CAD build for the part. Positions are in the model's coordinates, mm. A direction names the side the tool comes from. Round coordinates to 2 decimals unless told otherwise and drop trailing zeros. Write each loop counter-clockwise with the first axis right and the second up, starting at its lowest first coordinate (ties: lowest second). Pieces come first, ordered by that corner, then holes. Notation, with made-up numbers: (53, 41) -> (100, 41) arc R32 ccw to (100, 72) -> close; hole circle Ø11 at (-10.5, 42.25). An arc over 180 degrees is marked (long way). Put each result on its own line as item: value. Start each with the question number.
1. 3-axis set-ups, long thin cutter, end or side, ignore diameter. For faces 1 (the flat face through (1.014, -0.986, 1.724)), 2 (the cylindrical face through (0, 2, -1)): which of +Z, -Z, +X, -X, +Y, -Y reach the whole face in a straight line?
2. Saw through at A-A on z = -0.6. List the corners of the cut face in (x, y), and give its area (3 significant figures).
3. Saw through at B-B on y = -0.5. List the corners of the cut face in (x, z).
4. Saw through at D-D on y = 2.5. List the corners of the cut face in (x, z).
5. Saw through at C-C on x = 0.7. List the corners of the cut face in (y, z).
6. Drill centre lines: line 1 (Y direction, x = -1.65, z = 0.1); line 2 (X direction, y = 1.5, z = -0.5); line 3 (X direction, y = 0.25, z = 0). Where is each one in solid material? Low to high. Write a range as from..to.
7. Flat gauge pins, fed straight in: P1, Ø1, axis at x = -1, y = 4, coming from the +Z side; P2, Ø1, axis at x = -1.5, z = 1, coming from the +Y side; P3, Ø1.5, axis at x = -0.5, z = -1.5, coming from the +Y side. Where does each tip first touch, or does it go through?
from build123d import *

# Parameters (mm, degrees)
F0_R     = 1
F1_DEPTH = 2
F2_R     = 1
F3_DEPTH = 5
F4_DEPTH = 2


with BuildPart() as f1:
    # F0 (on Front) → F1 (new body)
    with BuildSketch(Plane.XZ):
        Polygon((-2, 1.1547005384), (-2, -1.1547005384), (0, -2.3094010768), (2, -1.1547005384), (2, 1.1547005384), (0, 2.3094010768), align=None)
        Circle(F0_R, mode=Mode.SUBTRACT)
        Circle(F0_R)
    extrude(amount=F1_DEPTH)

    # F2 (on face) → F3 (join)
    with BuildSketch(Plane(origin=(0, 0, 0), x_dir=(-1, 0, 0), z_dir=(0, 1, 0))):
        Circle(F2_R)
    extrude(amount=F3_DEPTH)

    # F0 (on Front) → F4 (join)
    with BuildSketch(Plane.XZ):
        Polygon((-2, 1.1547005384), (-2, -1.1547005384), (0, -2.3094010768), (2, -1.1547005384), (2, 1.1547005384), (0, 2.3094010768), align=None)
        Circle(F0_R, mode=Mode.SUBTRACT)
    extrude(amount=F4_DEPTH)


solid = f1.part
Return value:
1. face 1: +Z, +X, +Y, -Y
1. face 2: +Y
2. outline: (-2, -2) -> (2, -2) -> (2, 0) -> (0.8, 0) -> (0.8, 5) -> (-0.8, 5) -> (-0.8, 0) -> (-2, 0) -> close
2. area: 16.0 mm^2
3. outline: (-2, -1.15) -> (0, -2.31) -> (2, -1.15) -> (2, 1.15) -> (0, 2.31) -> (-2, 1.15) -> close
4. outline: circle Ø2 at (0, 0)
5. outline: (-2, -1.91) -> (0, -1.91) -> (0, -0.71) -> (5, -0.71) -> (5, 0.71) -> (0, 0.71) -> (0, 1.91) -> (-2, 1.91) -> close
6. line 1: y = -2..0
6. line 2: x = -0.87..0.87
6. line 3: x = -1..1
7. P1: stops at z = 0.87
7. P2: stops at y = 0
7. P3: stops at y = 5
